Build history of the part. All positions in model axes, mm. A direction names the side the tool comes from. Round coordinates to 2 decimals unless told otherwise and drop trailing zeros. Write each loop counter-clockwise with the first axis right and the second up, starting at its lowest first coordinate (ties: lowest second). Pieces come first, ordered by that corner, then holes. Notation, with made-up numbers: (47.5, 13) -> (95.5, 13) arc R5 ccw to (95.5, 20) -> close; hole circle Ø2 at (12.5, 7). An arc over 180 degrees is marked (long way). Answer in a Markdown table with one row per item.
Autodesk Inventor part; units mm, degrees
ref_plane "YZ Plane" through (0, 0, 0) normal (1, 0, 0) x (0, 1, 0)
ref_plane "XZ Plane" through (0, 0, 0) normal (0, 1, 0) x (-1, 0, 0)
ref_plane "XY Plane" through (0, 0, 0) normal (0, 0, 1) x (1, 0, 0)
sketch "Sketch1" plane through (0, 0, 0) normal (0, 1, 0) x (-1, 0, 0)
  line L0 (0, 0) -> (78.0034, 0)
  line L1 (78.0034, 0) -> (78.0034, -127.9906)
  line L2 (78.0034, -127.9906) -> (0, -127.9906)
  line L3 (0, -127.9906) -> (0, 0)
  dimension "d0" = 127.9906
  dimension "d1" = 78.0034
extrude "Extrusion1" add sketch "Sketch1" along normal blind 11.5062
sketch "Sketch2" plane through (0, 11.5062, 0) normal (0, 1, 0) x (1, 0, 0)
  line L0 (-78.0034, 0) -> (0, 0)
  line L1 (0, 127.9906) -> (-78.0034, 127.9906)
  line L2 (-39.0017, 0) -> (-39.0017, 127.9906) construction
  line L3 (-78.0034, 127.9906) -> (-78.0034, 0) construction
  line L4 (-78.0034, 63.9953) -> (0, 63.9953) construction
  line L5 (0, 0) -> (0, 127.9906) construction
  point P0 (-39.0017, 6.9977)
  point P1 (-39.0017, 120.9929)
  dimension "d4" = 113.9952
  dimension "d5" = 56.9976
hole "Hole1" at (-39.0017, 11.5062, -6.9977) at (-39.0017, 11.5062, -120.9929) direction (0, -1, 0) diameter 3.9878 depth 11.5062 counterbore diameter 7.112 counterbore depth 7.0612
sketch "Sketch3" plane through (0, 11.5062, 0) normal (0, 1, 0) x (1, 0, 0)
  line L0 (-73.9267, 14.4653) -> (-4.0767, 14.4653)
  line L1 (-4.0767, 14.4653) -> (-4.0767, 113.5253)
  line L2 (-4.0767, 113.5253) -> (-73.9267, 113.5253)
  line L3 (-73.9267, 113.5253) -> (-73.9267, 14.4653)
  line L4 (-78.0034, 0) -> (0, 0)
  line L5 (0, 0) -> (0, 127.9906)
  line L6 (0, 63.9953) -> (-78.0034, 63.9953) construction
  line L7 (-78.0034, 127.9906) -> (-78.0034, 0)
  line L8 (-39.0017, 0) -> (-39.0017, 127.9906) construction
  line L9 (0, 127.9906) -> (-78.0034, 127.9906)
  point P0 (-39.0017, 63.9953)
  dimension "d13" = 99.06
  dimension "d15" = 69.85
  dimension "d16" = 49.53
  dimension "d17" = 34.925
extrude "Extrusion2" add sketch "Sketch3" along normal blind 30.988 from surface at -11.5062 contours L3 L2 L1 L0
sketch "Sketch4" plane through (-73.9267, 30.988, -14.4653) normal (0, 1, 0) x (1, 0, 0)
  line L0 (30.8017, -0.4384) -> (30.8017, 99.4984) construction
  line L1 (30.8017, 99.4984) -> (42.6663, 99.4984) construction
  line L2 (42.6663, 99.4984) -> (42.6663, -0.4384) construction
  line L3 (42.6663, -0.4384) -> (30.8017, -0.4384) construction
  line L4 (69.85, 0) -> (0, 0)
  line L5 (0, 99.06) -> (69.85, 99.06)
  line L6 (0, 0) -> (0, 99.06)
  line L7 (69.85, 99.06) -> (69.85, 0)
  point P0 (73.9267, -14.4653)
properties part number "receiver box"
Q1. Wall check: line 1 (Z direction, x = -63.5, y = 13); line 2 (X direction, y = 12, z = -109.5); line 3 (Y direction, x = -33, z = -13). Give the ranges that are in metal, low to high. Write a range as [from, to].
A:
| item | result |
|---|---|
| line 1 | [-113.53, -14.47] |
| line 2 | [-73.93, -4.08] |
| line 3 | [0, 11.51] |
Q2. Saw through at C-C on y = 16. Write the cut outline in (x, z).
A:
| item | result |
|---|---|
| outline | (-73.93, -113.53) -> (-4.08, -113.53) -> (-4.08, -14.47) -> (-73.93, -14.47) -> close |
Q3. Saw through at B-B on z = -93.5. Write the cut outline in (x, y), plus the area to 3 significant figures.
A:
| item | result |
|---|---|
| outline | (-78, 0) -> (0, 0) -> (0, 11.51) -> (-4.08, 11.51) -> (-4.08, 30.99) -> (-73.93, 30.99) -> (-73.93, 11.51) -> (-78, 11.51) -> close |
| area | 2,260 mm² |
Q4. Which spindle directions (+Z, -Z, +X, -X, +Y, -Y) get a long thin tool onto all of the face, cutting with end or side? Do faces 4 (the flat face through (-39, 21, -14.465)), 5 (the flat face through (-73.927, 21, -65)), 6 (the flat face through (-39, 21, -113.525)), 7 (the cylindrical face through (-35.847, 7.926, -5.357)). Say none if no direction does.
A:
| item | result |
|---|---|
| face 4 | +Z, +X, -X, +Y |
| face 5 | +Z, -Z, -X, +Y |
| face 6 | -Z, +X, -X, +Y |
| face 7 | +Y |
Q5. Two-plate mould, pull along X, no slides. Class faces 1 (the flat face through (-4.077, 21, -63)), 2 (the cylindrical face through (-37.64, 7.93, -117.71)), 3 (the flat face through (-38, 6, 0)): released by +X, released by -X, zero draft, split by the parting line, or undercut.
A:
| item | result |
|---|---|
| face 1 | released by +X |
| face 2 | undercut |
| face 3 | zero draft |
Q6. Saw through at A-A on x = -14. Write the cut outline in (y, z).
A:
| item | result |
|---|---|
| outline | (0, -127.99) -> (11.51, -127.99) -> (11.51, -113.53) -> (30.99, -113.53) -> (30.99, -14.47) -> (11.51, -14.47) -> (11.51, 0) -> (0, 0) -> close |
Q7. Drop flat-ended pins along their axis: P1, Ø3.5, axis at x = -40.5, z = -6.5, coming from the +Y side (3 decimals); P2, Ø1.5, axis at x = -37, z = -71.5, coming from the -Y side; P3, Ø1.5, axis at y = 24.5, z = -65.5, coming from the -X side; P4, Ø4, axis at x = -42.5, y = 22.5, coming from the -Z side. Give the stop position or say it passes through.
A:
| item | result |
|---|---|
| P1 | y = 4.445 |
| P2 | y = 0 |
| P3 | x = -73.93 |
| P4 | z = -113.53 |
